Part model, mm, in its own coordinate system. A direction names the side the tool comes from. Round coordinates to 2 decimals unless told otherwise and drop trailing zeros. Write each loop counter-clockwise with the first axis right and the second up, starting at its lowest first coordinate (ties: lowest second). Pieces come first, ordered by that corner, then holes. Notation, with made-up numbers: M 69,18.5 L 74,18.5 A29 cw 74,44.5 Z; hole C -3,-32 d7. An arc over 180 degrees is marked long. Use a Markdown table: item, result. Add a question column.
1) Slice it at B-B on y = -7.5. Write the cut outline in (x, z), plus the area to 3 significant figures.
2) Two-plate mould, pull along Z, no slides. Class faces 4 (the face through (7.075, 54.246, 8.698)), 5 (the face through (22.76, 54.41, 8.7)), 6 (the face through (34, 27, 25)), 7 (the face through (31.972, 36.276, 21.996)): released by +Z, released by -Z, zero draft, split by the parting line, or undercut.
3) Drop flat-ended pins along their axis: P1, Ø8, axis at y = 52.5, z = 7, coming from the +X side; P2, Ø4, axis at x = 6, y = 54, coming from the +Z side; P3, Ø4, axis at y = 11.5, z = 4.5, coming from the -X side. Give the stop position or say it passes through.
4) Which spindle directions (+Z, -Z, +X, -X, +Y, -Y) get a long thin tool onto all of the face, cutting with end or side? Do faces 1 (the face through (15, 4, 25)), 2 (the face through (-1.97, 33.82, 18.24)), 3 (the face through (-4, 27, 25)). Say none if no direction does.
5) Wall check: probe 1 along X at (y, z) = (-19, 8); probe 2 along Z at (x, y) = (9, -28); probe 3 along Z at (x, y) = (1, -3). Give the ranges that are in metal, low to high.
6) Slice it at A-A on z = 32. Write the cut outline in (x, y), plus the area to 3 significant figures.
Autodesk Fusion 360 part; units mm, degrees
sketch "Sketch1" plane through (0, 0, 0) normal (0, 0, 1) x (1, 0, 0)
sketch "Sketch2" plane through (0, 0, 0) normal (0, 0, 1) x (1, 0, 0)
sketch "Sketch3" plane through (0, 0, 0) normal (0, 0, 1) x (1, 0, 0)
  line L0 (0, 0) -> (0, 50)
  line L1 (0, 50) -> (15, 65)
  line L2 (15, 65) -> (30, 50)
  line L3 (30, 50) -> (30, 0)
  line L4 (30, 0) -> (0, 0)
extrude "Extrude1" add sketch "Sketch3" along normal blind 25
fillet "Fillet1" radius 12.5 2 edges at (22.5, 57.5, 25) (7.5, 57.5, 25)
fillet "Fillet2" radius 5 4 edges at (0, 25, 0) (30, 25, 0) (22.5, 57.5, 0) (7.5, 57.5, 0)
fillet "Fillet3" radius 5 3 edges at (15, 62.9289, 1.4645) (15, 65, 8.75) (15, 59.8223, 21.3388)
extrude "Extrude2" add 1 faces at (11.6667, 0, 16.6667) along direction (0, -1, 0) blind 40
extrude "Extrude3" cut 1 faces at (22.3452, 57.6548, 10) along direction (-0.707107, -0.707107, 0) blind 2
extrude "Extrude4" cut 1 faces at (7.6548, 57.6548, 10) along direction (0.707107, -0.707107, 0) blind 2
sketch "Sketch4" plane through (0, 0, 0) normal (-1, 0, 0) x (0, -1, 0)
  line L0 (-50, 5) -> (40, 5)
  line L1 (40, 5) -> (40, 25)
  line L2 (40, 25) -> (-32.3223, 25)
  ellipse E0 centre (-32.3223, 12.5) end of major axis (-50, 12.5) minor radius 12.5 (-32.3223, 25) -> (-50, 12.5) ccw
  line L3 (-50, 12.5) -> (-50, 5)
  circle A0 centre (-26.4534, 25) radius 10
  dimension "d15" = 20
extrude "Extrude5" add sketch "Sketch4" along normal blind 3 contours L2 E0 A0 | L2 E0 A0
extrude "Extrude6" add 1 faces at (-3, 25.7282, 28.0287) along direction (-1, 0, 0) blind 1
sketch "Sketch5" plane through (30, 0, 0) normal (1, 0, 0) x (0, 1, 0)
  line L0 (-40, 5) -> (50, 5)
  line L1 (50, 5) -> (50, 12.5)
  ellipse E0 centre (32.3223, 12.5) end of major axis (50, 12.5) minor radius 12.5 (50, 12.5) -> (32.3223, 25) ccw
  line L2 (32.3223, 25) -> (-40, 25)
  line L3 (-40, 25) -> (-40, 5)
  circle A0 centre (26.7382, 25) radius 10
  dimension "d20" = 20
extrude "Extrude7" add sketch "Sketch5" along normal blind 4 contours E0 L2 A0 | E0 L2 A0
Entries:
| question | item | result |
|---|---|---|
| 1 | outline | M 0,5 A5 ccw 5,0 L 25,0 A5 ccw 30,5 L 30,25 L 0,25 Z |
| 1 | area | 739 mm^2 |
| 2 | face 4 | undercut |
| 2 | face 5 | undercut |
| 2 | face 6 | zero draft |
| 2 | face 7 | split by the parting line |
| 3 | P1 | stops at x = 30 |
| 3 | P2 | stops at z = 21.08 |
| 3 | P3 | stops at x = 0 |
| 4 | face 1 | +Z, +Y, -Y |
| 4 | face 2 | -X |
| 4 | face 3 | +Z, -Z, -X, +Y, -Y |
| 5 | probe 1 | x = 0 to 30 |
| 5 | probe 2 | z = 0 to 25 |
| 5 | probe 3 | z = 2 to 25 |
| 6 | outline | M -4,19.31 L 0,19.31 L 0,33.59 L -4,33.59 Z; M 30,19.6 L 34,19.6 L 34,33.88 L 30,33.88 Z |
| 6 | area | 114 mm^2 |
